Build history of the part. All positions in model axes, mm. A direction names the side the tool comes from. Round coordinates to 2 decimals unless told otherwise and drop trailing zeros. Loops run counter-clockwise (first coordinate to the right, second up) from the corner with the lowest first, then second, coordinate; pieces in that order, holes last. Notation, with made-up numbers: (-14, 13) - (-10, 13) arc R19 ccw to (-10, 47) - close; hole circle Ø1 at (45, 72). An arc over 180 degrees is marked (long way). Put each result on its own line as item: value. Start each with the question number.
from build123d import *

# Parameters (mm, degrees)
F0_W         = 32
F0_H         = 20
F1_DEPTH     = 1.5
F2_DEPTH     = 11
F3_DEPTH     = 5
F4_R         = 2
F5_T1_DEPTH  = 15
F5_S5_W      = 2.04
F5_S5_H      = 2.04
F5_T6_DEPTH  = 2.04
F5_S11_W     = 2.04
F5_S11_H     = 2.04
F5_T12_DEPTH = 2.04


# Not quite as in the source:
# - a fillet or chamfer that OpenCascade refuses, or shapes differently, is made with other operations: its cross-section is extruded or revolved along the edge and cut away or added


with BuildPart() as f1:
    # F0 (on Front) → F1 (new body)
    with BuildSketch(Plane.XZ):
        with Locations((0.460526906, 4.9254382253)):
            Rectangle(F0_W, F0_H)
    extrude(amount=F1_DEPTH)

    # F0 (on Front) → F2 (join)
    with BuildSketch(Plane.XZ):
        Polygon((-15.539473094, -5.0745617747), (-15.539473094, 14.9254382253), (16.460526906, 14.9254382253), (16.460526906, -5.0745617747), (17.960526906, -5.0745617747), (17.960526906, 16.4254382253), (-17.039473094, 16.4254382253), (-17.039473094, -5.0745617747), align=None)
    extrude(amount=F2_DEPTH)

    # F0 (on Front) → F3 (join)
    with BuildSketch(Plane.XZ):
        Polygon((16.460526906, -5.0745617747), (-15.539473094, -5.0745617747), (-17.039473094, -5.0745617747), (-17.039473094, -6.5745617747), (17.960526906, -6.5745617747), (17.960526906, -5.0745617747), align=None)
    extrude(amount=F3_DEPTH)

    # F4
    f4_edges = [f1.edges().sort_by_distance(p)[0] for p in [
        (17.960527, 0, 4.925438),
        (0.460527, 0, 16.425438),
        (-17.039473, 0, 4.925438),
        (0.460527, 0, -6.574562),
        (17.960527, -5.5, 16.425438),
        (-17.039473, -5.5, 16.425438),
    ]]
    fillet(f4_edges, radius=F4_R)

    # F5: fillet of radius 2 on 2 edges, made by hand

    # F5_s2 → F5_t1 (cut)
    with BuildSketch(Plane.XZ.offset(2)):
        with BuildLine():
            ThreePointArc((-17.039473094, -4.5745617747), (-16.4536866564, -5.9887753371), (-15.039473094, -6.5745617747))
            Line((-15.039473094, -6.5745617747), (-15.039473094, -6.6145617747))
            Line((-15.039473094, -6.6145617747), (-17.079473094, -6.6145617747))
            Line((-17.079473094, -6.6145617747), (-17.079473094, -4.5745617747))
            Line((-17.079473094, -4.5745617747), (-17.039473094, -4.5745617747))
        make_face()
        with BuildLine():
            ThreePointArc((15.960526906, -6.5745617747), (17.3747404683, -5.9887753371), (17.960526906, -4.5745617747))
            Line((17.960526906, -4.5745617747), (18.000526906, -4.5745617747))
            Line((18.000526906, -4.5745617747), (18.000526906, -6.6145617747))
            Line((18.000526906, -6.6145617747), (15.960526906, -6.6145617747))
            Line((15.960526906, -6.6145617747), (15.960526906, -6.5745617747))
        make_face()
    extrude(amount=F5_T1_DEPTH, mode=Mode.SUBTRACT)


with BuildPart() as f5_tool4:
    # F5_s5 → F5_t6 (new body)
    with BuildSketch(Plane.XY.offset(-4.5745617747)):
        with Locations((16.980526906, -0.98)):
            Rectangle(F5_S5_W, F5_S5_H)
    extrude(amount=-F5_T6_DEPTH)

    # F5_s7 → F5_t8 (revolve, cut)
    with BuildSketch(Plane(origin=(15.960526906, -2, -4.5745617747), x_dir=(-0.7071067812, -0.7071067812, 0), z_dir=(0.7071067812, -0.7071067812, 0))):
        with BuildLine():
            ThreePointArc((0, -2), (2, 0), (0, 2))
            Line((0, 2), (0, -2))
        make_face()
    revolve(axis=Axis((15.960526906, -2, -4.5745617747), (0, 0, -1)), mode=Mode.SUBTRACT)


with BuildPart() as f1_1:
    add(f1.part)

    # F5_t3: cut F5_tool4
    add(f5_tool4.part, mode=Mode.SUBTRACT)


with BuildPart() as f5_tool10:
    # F5_s11 → F5_t12 (new body)
    with BuildSketch(Plane.YZ.offset(-15.039473094)):
        with Locations((-0.98, -5.5945617747)):
            Rectangle(F5_S11_W, F5_S11_H)
    extrude(amount=-F5_T12_DEPTH)

    # F5_s13 → F5_t14 (revolve, cut)
    with BuildSketch(Plane(origin=(-15.039473094, -2, -4.5745617747), x_dir=(0, -0.7071067812, 0.7071067812), z_dir=(0, -0.7071067812, -0.7071067812))):
        with BuildLine():
            ThreePointArc((0, -2), (2, 0), (0, 2))
            Line((0, 2), (0, -2))
        make_face()
    revolve(axis=Axis((-15.039473094, -2, -4.5745617747), (-1, 0, 0)), mode=Mode.SUBTRACT)


with BuildPart() as f1_2:
    add(f1_1.part)

    # F5_t9: cut F5_tool10
    add(f5_tool10.part, mode=Mode.SUBTRACT)


solid = f1_2.part
Item 1: Which spindle directions (+Z, -Z, +X, -X, +Y, -Y) get a long thin tool onto all of the face, cutting with end or side? Do faces 1 (the flat face through (1, -3, -5.075)), 2 (the cylindrical face through (-16.469, -6.563, 15.824)), 3 (the flat face through (17, -8, -5.075)). Say none if no direction does.
Item 2: Drop flat-ended pins along their axis: pin 1 Ø1.6 at (x, y) = (17, -7.5) entering from -Z; pin 2 Ø6 at (x, z) = (-7.5, 8) entering from -Y; pin 3 Ø1.7 at (x, z) = (5, -5.5) entering from -Y. Give the stop position or say it passes through.
Item 3: Slice it at B-B (z = 9.5). Give the cut face in (x, y), plus the area to 3 significant figures.
Item 4: Slice it at A-A (y = -3.25). Give the cut face in (x, z), plus the area to 3 significant figures.
Item 5: Two-plate mould, pull along X, no slides. Class faces 4 (the flat face through (17.961, -6, 5)), 5 (the cylindrical face through (-16.47, -0.6, 4.79)), 6 (the flat face through (16.461, -6, 5)): pulls with the +X half, pulls with the -X half, needs draft (parallel to the pull), parting line crosses it, or undercut.
Item 6: Slice it at C-C (x = 3). Give the cut face in (y, z), plus the area to 3 significant figures.
Item 7: Slice it at D-D (y = -9.75). Give the cut face in (x, z).
Item 8: Drill centre lines: probe 1 along X at (y, z) = (-8.5, 12.5); probe 2 along Z at (x, y) = (-9, -4.25); probe 3 along Y at (x, z) = (10.5, -3.75). Where is each one in solid material? Low to high. Write a range as [from, to].
Computed values:
1. face 1: -Y
1. face 2: +Z, -X, +Y, -Y
1. face 3: -Z, +X, -X, -Y
2. pin 1: stops at z = -5.07
2. pin 2: stops at y = -1.5
2. pin 3: stops at y = -5
3. outline: (-17.04, -11) - (-15.54, -11) - (-15.54, -1.5) - (16.46, -1.5) - (16.46, -11) - (17.96, -11) - (17.96, -2) arc R2 ccw to (15.96, 0) - (-15.04, 0) arc R2 ccw to (-17.04, -2) - close
3. area: 79.3 mm^2
4. outline: (-17.04, -4.57) arc R2 ccw to (-15.04, -6.57) - (15.96, -6.57) arc R2 ccw to (17.96, -4.57) - (17.96, 14.43) arc R2 ccw to (15.96, 16.43) - (-15.04, 16.43) arc R2 ccw to (-17.04, 14.43) - close; hole (-15.54, -5.07) - (16.46, -5.07) - (16.46, 14.93) - (-15.54, 14.93) - close
4. area: 162 mm^2
5. face 4: pulls with the +X half
5. face 5: pulls with the -X half
5. face 6: undercut
6. outline: (-11, 14.93) - (-1.5, 14.93) - (-1.5, -5.07) - (-5, -5.07) - (-5, -6.57) - (-2, -6.57) arc R2 ccw to (0, -4.57) - (0, 14.43) arc R2 ccw to (-2, 16.43) - (-11, 16.43) - close
6. area: 52.3 mm^2
7. outline: (-17.04, -4.57) arc R2 ccw to (-16.98, -5.07) - (-15.54, -5.07) - (-15.54, 14.93) - (16.46, 14.93) - (16.46, -5.07) - (17.9, -5.07) arc R2 ccw to (17.96, -4.57) - (17.96, 14.43) arc R2 ccw to (15.96, 16.43) - (-15.04, 16.43) arc R2 ccw to (-17.04, 14.43) - close
8. probe 1: x = [-17.04, -15.54], [16.46, 17.96]
8. probe 2: z = [-6.57, -5.07], [14.93, 16.43]
8. probe 3: y = [-1.5, 0]
